Build history of the part. All positions in model axes, mm. Round coordinates to 2 decimals unless told otherwise and drop trailing zeros. Loops run counter-clockwise (first coordinate to the right, second up) from the corner with the lowest first, then second, coordinate; pieces in that order, holes last. Notation, with made-up numbers: (31.5, 83.5) - (71.5, 83.5) arc R31 ccw to (71.5, 110.5) - close; hole circle Ø5 at (49.25, -16). An arc over 180 degrees is marked (long way). Answer as CSV lines item,"result". Start each with the question number.
```python
from build123d import *

# Parameters (mm, degrees)
EXTRUDE_1_DEPTH          = 3
SKETCH_2_R               = 5
CUT_EXTRUDE_1_DEPTH      = 3
SKETCH_3_R               = 1.2
CUT_EXTRUDE_2_DEPTH      = 3
PATTERN_CIRCULAR_1_COUNT = 3


with BuildPart() as part:
    # 草图1 → 凸台-拉伸1 (new body)
    with BuildSketch(Plane(origin=(0, 0, 0), x_dir=(1, 0, 0), z_dir=(0, 1, 0))):
        Polygon((28.867513459, 50), (-28.867513459, 50), (-57.735026919, 0), (-28.867513459, -50), (28.867513459, -50), (57.735026919, 0), align=None)
    extrude(amount=EXTRUDE_1_DEPTH)

    # 草图2 → 切除-拉伸1 (cut)
    with BuildSketch(Plane(origin=(0, 3, 0), x_dir=(1, 0, 0), z_dir=(0, 1, 0))):
        with Locations(Location((0, 0, 0), (0, 0, 270))):
            Circle(SKETCH_2_R)
    extrude(amount=-CUT_EXTRUDE_1_DEPTH, mode=Mode.SUBTRACT)

    # 草图3 → 切除-拉伸2 (cut)
    with BuildSketch(Plane.XZ):
        with Locations(Location((-8, 45, 0), (0, 0, 270))):
            Circle(SKETCH_3_R)
        with Locations(Location((8, 45, 0), (0, 0, 270))):
            Circle(SKETCH_3_R)
        with Locations(Location((8, 35, 0), (0, 0, 270))):
            Circle(SKETCH_3_R)
        with Locations(Location((-8, 35, 0), (0, 0, 270))):
            Circle(SKETCH_3_R)
    cut_extrude_2 = extrude(amount=-CUT_EXTRUDE_2_DEPTH, mode=Mode.SUBTRACT)

    # 阵列(圆周)1: 切除-拉伸2 ×3 about axis
    pattern_circular_1_axis = Axis((0, 0, 0), (0, 1, 0))
    for i in range(1, PATTERN_CIRCULAR_1_COUNT):
        add(cut_extrude_2.rotate(pattern_circular_1_axis, i * 360 / PATTERN_CIRCULAR_1_COUNT), mode=Mode.SUBTRACT)


solid = part.part
```
Q1. Pin check, flat tips, straight feed: pin 1 Ø3 at (x, z) = (34.31, -10.57) entering from +Y; pin 2 Ø1 at (y, z) = (2.5, 4.5) entering from +X. Stop position of each tip, or through.
Q2. Band-saw the part on C-C, the plane x = -31. List the corners of the cut face in (y, z).
Q3. Wall check: probe 1 along X at (y, z) = (2.25, 45); probe 2 along X at (y, z) = (2.8, 35.5); probe 3 along X at (y, z) = (1, 0). Give the ranges that are in metal, low to high. Write a range as [from, to].
Q4. Band-saw the part on A-A, the plane y = 0.6. Give the number of separate pieces and of enclosed holes in the cut face, then the cut area to 3 significant figures.
Q5. Band-saw the part on B-B, the plane z = 23. List the corners of the cut face in (x, y), then the cut area to 3 significant figures.
Q6. Two-plate mould, pull along X, no slides. Class faces 1 (the flat face through (43.1, 1.48, 25.35)), 2 (the cylindrical face through (-4.88, 1.52, -1.08)), 3 (the flat face through (12, 0, -1)): released by +X, released by -X, zero draft, split by the parting line, or undercut.
Reported:
1,pin 1,"stops at y = 3"
1,pin 2,"stops at x = 55.43"
2,outline,"(0, -46.31) - (3, -46.31) - (3, 46.31) - (0, 46.31) - close"
3,probe 1,"x = [-31.75, -9.2], [-6.8, 6.8], [9.2, 31.75]"
3,probe 2,"x = [-37.24, -9.09], [-6.91, 6.91], [9.09, 37.24]"
3,probe 3,"x = [-57.74, -5], [5, 57.74]"
4,separate pieces,"1"
4,enclosed holes,"13"
4,area,"8,530 mm2"
5,outline,"(-44.46, 0) - (44.46, 0) - (44.46, 3) - (-44.46, 3) - close"
5,area,"267 mm2"
6,face 1,"released by +X"
6,face 2,"undercut"
6,face 3,"zero draft"
